Autodesk Fusion 360 part; units mm, degrees
sketch "Esquisse1" plane through (0, 0, 0) normal (0, 0, 1) x (1, 0, 0)
  line L0 (0, 0) -> (2.4, 0)
  line L1 (2.4, 0) -> (2.4, 1.2)
  line L2 (2.4, 1.2) -> (0, 1.2)
  line L3 (0, 1.2) -> (0, 0)
  dimension "d1" = 2.4
  dimension "d2" = 1.2
extrude "Extrusion1" add sketch "Esquisse1" along normal blind 1
sketch "Esquisse2" plane through (2.4, 0, 0) normal (1, 0, 0) x (0, 1, 0)
  line L0 (0, 0) -> (1.2, 0)
  line L1 (1.2, 0) -> (1.2, 1)
  line L2 (1.2, 1) -> (0, 1)
  line L3 (0, 1) -> (0, 0)
  circle A0 centre (0.6, 0.5) radius 0.125
  dimension "d5" = 0.25
extrude "Extrusion2" add sketch "Esquisse2" along normal blind 1 contours A0
scale "Echelle1" factor 10 about (0, 1.2, 1) bodies 1
Verification items for the finished model (mm, model axes). A direction names the side the tool comes from. Round coordinates to 2 decimals unless told otherwise and drop trailing zeros. Write each loop counter-clockwise with the first axis right and the second up, starting at its lowest first coordinate (ties: lowest second). Pieces come first, ordered by that corner, then holes.
1. Section check D-D on z = -7.5. Enter the section's corners in (x, y), plus the area to 3 significant figures.
2. Section check A-A on y = -4.8. Enter the section's corners in (x, z).
3. Gauge pin test, flat ends, axial feed: P1, Ø4, axis at y = -8, z = -6, coming from the +X side; P2, Ø6, axis at x = 30.5, y = -2.5, coming from the -Z side. Record the tip position at first contact, or that the pin passes through.
4. Section check B-B on z = -4. Enter the section's corners in (x, y), plus the area to 3 significant figures.
5. Access from +Z, -Z, +X, -X, +Y, -Y to the whole of each face (thin tool, end or side, straight path). Record for faces 1 (the flat face through (0, -5, -4)), 2 (the cylindrical face through (28.93, -5.07, -2.78)).
6. Section check C-C on x = 25.5. Enter the section's corners in (y, z), plus the area to 3 significant figures.
7. Scan lines: L1, parallel to X at y = -10, z = -6; L2, parallel to Y at x = 29, z = -3.75; L3, parallel to Y at x = 31, z = -4.75. Record each from-to range of solid material in increasing order.
Answer:
1. outline: (0, -10.8) - (24, -10.8) - (24, 1.2) - (0, 1.2) - close
1. area: 288 mm2
2. outline: (0, -9) - (24, -9) - (24, -5.25) - (34, -5.25) - (34, -2.75) - (24, -2.75) - (24, 1) - (0, 1) - close
3. P1: stops at x = 24
3. P2: stops at z = -5.25
4. outline: (0, -10.8) - (24, -10.8) - (24, -6.05) - (34, -6.05) - (34, -3.55) - (24, -3.55) - (24, 1.2) - (0, 1.2) - close
4. area: 313 mm2
5. face 1: +Z, -Z, -X, +Y, -Y
5. face 2: +X
6. outline: circle Ø2.5 at (-4.8, -4)
6. area: 4.91 mm2
7. L1: x = 0 to 24
7. L2: y = -6.02 to -3.58
7. L3: y = -5.8 to -3.8
